The listing builds one solid part. Answer for the finished solid, in the listing's coordinates (mm). Give positions to 0.01 mm unless a question says otherwise; leave off trailing zeros. Order: outer loops, then holes, each group sorted by start corner. A loop starts at its lowest first (then second) coordinate and runs counter-clockwise, first axis right, second up.
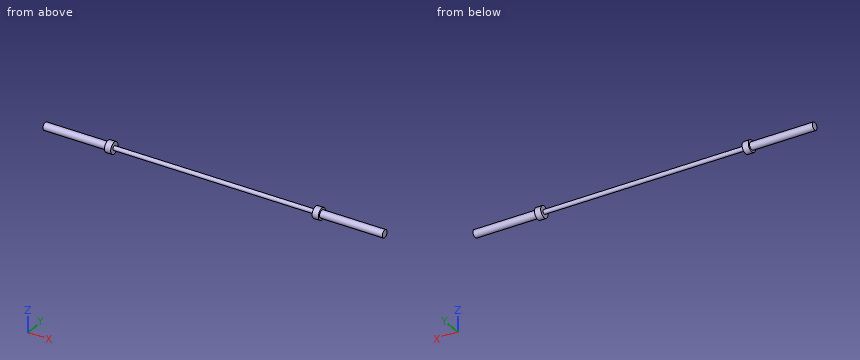
```python
from build123d import *

# Parameters (mm, degrees)
F0_R     = 25
F1_DEPTH = 415
F2_R     = 38.1
F3_DEPTH = 41.275
F4_R     = 14
F5_DEPTH = 1333.5
F6_R     = 38.1
F7_DEPTH = 41.275
F8_R     = 25
F9_DEPTH = 415


with BuildPart() as f1:
    # F0 (on Right) → F1 (new body)
    with BuildSketch(Plane.YZ):
        Circle(F0_R)
    extrude(amount=-F1_DEPTH)



with BuildPart() as f3:
    # F2 (on face) → F3 (new body)
    with BuildSketch(Plane(origin=(-1789.775, 0, 0), x_dir=(0, -1, 0), z_dir=(-1, 0, 0))):
        Circle(F2_R)
    extrude(amount=F3_DEPTH)

    # F4 (on face) → F5 (join)
    with BuildSketch(Plane(origin=(-456.275, 0, 0), x_dir=(0, -1, 0), z_dir=(-1, 0, 0))):
        Circle(F4_R)
    extrude(amount=F5_DEPTH)


with BuildPart() as f1_1:
    add(f1.part)

    add(f3.part)  # F7 merges F3
    # F6 (on face) → F7 (join)
    with BuildSketch(Plane(origin=(-415, 0, 0), x_dir=(0, -1, 0), z_dir=(-1, 0, 0))):
        Circle(F6_R)
    extrude(amount=F7_DEPTH)

    # F8 (on face) → F9 (join)
    with BuildSketch(Plane(origin=(-1831.05, 0, 0), x_dir=(0, -1, 0), z_dir=(-1, 0, 0))):
        Circle(F8_R)
    extrude(amount=F9_DEPTH)


solid = f1_1.part
```
1) Straight lines are drawn through the part: probe 1 along X at (y, z) = (-16, 32) (3 decimals); probe 2 along X at (y, z) = (-14.5, 16) (3 decimals); probe 3 along Y at (x, z) = (-1194, -3.5). For each, find the intervals that lie inside material, in ascending order.
Geometry says:
probe 1: x = -1831.05 to -1789.775, -456.275 to -415
probe 2: x = -2246.05 to -1789.775, -456.275 to 0
probe 3: y = -13.56 to 13.56
2) Find section A-A (z = 0). Write down the section's boundary in (x, y) (3 decimals).
Geometry says:
outline: (-2246.05, -25) - (-1831.05, -25) - (-1831.05, -38.1) - (-1789.775, -38.1) - (-1789.775, -14) - (-456.275, -14) - (-456.275, -38.1) - (-415, -38.1) - (-415, -25) - (0, -25) - (0, 25) - (-415, 25) - (-415, 38.1) - (-456.275, 38.1) - (-456.275, 14) - (-1789.775, 14) - (-1789.775, 38.1) - (-1831.05, 38.1) - (-1831.05, 25) - (-2246.05, 25) - close
3) Given P1, Ø6, axis at x = -1165, y = 15.5, coming from the +Z side; P2, Ø8, axis at y = -3, z = -30.5, coming from the -X side; P3, Ø3, axis at x = -1846.5, z = 21.5, coming from the +Y side, each flat-ended and moving along its own axis, determine where each tip first touches the part or whether it passes through.
Geometry says:
P1: stops at z = 6.3
P2: stops at x = -1831.05
P3: stops at y = 15
4) Find section C-C (x = -517). Write down the section's boundary in (y, z), then the cut area to 3 significant figures.
Geometry says:
outline: circle Ø28 at (0, 0)
area: 616 mm2
